Input: part model. Units: mm. Frame: model coordinates. A direction names the side the tool comes from. Coordinates: 2 decimals unless noted, no trailing zeros. Write each loop counter-clockwise with the first axis right and the second up, starting at its lowest first coordinate (ties: lowest second). Pieces come first, ordered by that corner, then holes. Notation, with made-up numbers: M -6,69.25 L 46,69.25 A31 cw 46,107.25 Z; hole C 32.5,80.25 d3. An arc over 180 degrees is marked long. Use one line per item in the form item = value.
from build123d import *

# Parameters (mm, degrees)
F0_W      = 30.5
F0_H      = 22.5
F1_DEPTH  = 6.5
F3_DEPTH  = 3
F4_W      = 7
F4_H      = 4.5
F5_DEPTH  = 3
F6_W      = 6.5
F6_H      = 2.5
F7_DEPTH  = 3.75
F8_W      = 5.8
F8_H      = 1.5
F9_DEPTH  = 0.5
F11_DEPTH = 1
F13_DEPTH = 2.5
F14_W     = 0.5
F14_H     = 0.25
F15_DEPTH = 7
F16_W     = 21.5
F16_H     = 5.5
F17_DEPTH = 1


with BuildPart() as f1:
    # F0 (on Top) → F1 (new body)
    with BuildSketch(Plane.XY):
        Rectangle(F0_W, F0_H)
    extrude(amount=F1_DEPTH)

    # F2 (on face) → F3 (cut)
    with BuildSketch(Plane.XY.offset(6.5)):
        with BuildLine():
            Line((-7.25, 11.25), (-15.25, 11.25))
            Line((-15.25, 11.25), (-15.25, 6.25))
            Line((-15.25, 6.25), (-8.25, 6.25))
            ThreePointArc((-8.25, 6.25), (-7.542893, 6.542893), (-7.25, 7.25))
            Line((-7.25, 7.25), (-7.25, 11.25))
        make_face()
    extrude(amount=-F3_DEPTH, mode=Mode.SUBTRACT)

    # F4 (on face) → F5 (join)
    with BuildSketch(Plane.XY.offset(3.5)):
        with Locations((-11.75, 9)):
            Rectangle(F4_W, F4_H)
    extrude(amount=F5_DEPTH)

    # F6 (on face) → F7 (cut)
    with BuildSketch(Plane(origin=(0, 11.25, 0), x_dir=(-1, 0, 0), z_dir=(0, 1, 0))):
        with Locations((11.75, 5)):
            Rectangle(F6_W, F6_H)
    extrude(amount=-F7_DEPTH, mode=Mode.SUBTRACT)

    # F8 (on face) → F9 (cut)
    with BuildSketch(Plane.XY.offset(6.5)):
        with Locations((-11.75, 10.5)):
            Rectangle(F8_W, F8_H)
    extrude(amount=-F9_DEPTH, mode=Mode.SUBTRACT)

    # F10 (on face) → F11 (cut)
    with BuildSketch(Plane.XY.offset(6.5)):
        with BuildLine():
            Line((10.25, 11.25), (1.75, 11.25))
            Line((1.75, 11.25), (1.75, 8.25))
            ThreePointArc((1.75, 8.25), (2.042893, 7.542893), (2.75, 7.25))
            Line((2.75, 7.25), (9.25, 7.25))
            ThreePointArc((9.25, 7.25), (9.957107, 7.542893), (10.25, 8.25))
            Line((10.25, 8.25), (10.25, 11.25))
        make_face()
    extrude(amount=-F11_DEPTH, mode=Mode.SUBTRACT)

    # F12 (on face) → F13 (join)
    with BuildSketch(Plane(origin=(-15.25, 0, 0), x_dir=(0, -1, 0), z_dir=(-1, 0, 0))):
        with BuildLine():
            Line((10.75, 6.5), (-3.25, 6.5))
            ThreePointArc((-3.25, 6.5), (-3.603553, 6.353553), (-3.75, 6))
            Line((-3.75, 6), (-3.75, 2))
            ThreePointArc((-3.75, 2), (-3.603553, 1.646447), (-3.25, 1.5))
            Line((-3.25, 1.5), (10.75, 1.5))
            ThreePointArc((10.75, 1.5), (11.103553, 1.646447), (11.25, 2))
            Line((11.25, 2), (11.25, 6))
            ThreePointArc((11.25, 6), (11.103553, 6.353553), (10.75, 6.5))
        make_face()
    extrude(amount=F13_DEPTH)

    # F14 (on face) → F15 (join)
    with BuildSketch(Plane(origin=(-17.75, 0, 0), x_dir=(0, -1, 0), z_dir=(-1, 0, 0))):
        with Locations((-2.5, 5.5)):
            Rectangle(F14_W, F14_H)
        with Locations((-2.5, 2.5)):
            Rectangle(F14_W, F14_H)
        with Locations((0, 5.5)):
            Rectangle(F14_W, F14_H)
        with Locations((0, 2.5)):
            Rectangle(F14_W, F14_H)
        with Locations((2.5, 5.5)):
            Rectangle(F14_W, F14_H)
        with Locations((2.5, 2.5)):
            Rectangle(F14_W, F14_H)
        with Locations((5, 5.5)):
            Rectangle(F14_W, F14_H)
        with Locations((5, 2.5)):
            Rectangle(F14_W, F14_H)
        with Locations((7.5, 5.5)):
            Rectangle(F14_W, F14_H)
        with Locations((7.5, 2.5)):
            Rectangle(F14_W, F14_H)
        with Locations((10, 5.5)):
            Rectangle(F14_W, F14_H)
        with Locations((10, 2.5)):
            Rectangle(F14_W, F14_H)
    extrude(amount=F15_DEPTH)

    # F16 (on face) → F17 (cut)
    with BuildSketch(Plane.YZ.offset(15.25)):
        with Locations((0, 3.25)):
            Rectangle(F16_W, F16_H)
    extrude(amount=-F17_DEPTH, mode=Mode.SUBTRACT)


solid = f1.part
(1) First-contact query: pin 1 Ø5 at (x, y) = (-19.5, 4.5) entering from -Z; pin 2 Ø0.8 at (y, z) = (8.5, 5) entering from -X; pin 3 Ø0.6 at (x, y) = (-22.5, -7.5) entering from -Z (3 decimals). Flat tips, straight axial feed; report the tip coordinate or a pass-through.
Computed:
pin_1 = 1.5
pin_2 = -15.25
pin_3 = 2.375
(2) Section query B-B on y = -3.5. Return the cut outline in (x, z).
Computed:
outline = M -17.75,1.5 L -15.25,1.5 L -15.25,0 L 15.25,0 L 15.25,0.5 L 14.25,0.5 L 14.25,6 L 15.25,6 L 15.25,6.5 L -17.75,6.5 Z
(3) Pull-direction query (X, two-part tool) for faces 6 (the flat face through (15, 10.75, 3)), 7 (the flat face through (-7.25, 9, 5)); classes: pulls with the +X half, pulls with the -X half, needs draft (parallel to the pull), parting line crosses it, or undercut.
Computed:
face_6 = needs draft
face_7 = undercut
(4) Line query: probe 1 along Y at (x, z) = (-22, 5.5); probe 2 along X at (y, z) = (7.75, 5.75); probe 3 along X at (y, z) = (-8.5, 1). Output: solid intervals per line, ascending.
Computed:
probe_1 = -10.25 to -9.75, -7.75 to -7.25, -5.25 to -4.75, -2.75 to -2.25, -0.25 to 0.25, 2.25 to 2.75
probe_2 = -15.25 to -15, -8.5 to -8.25, -7.25 to 1.88, 10.12 to 14.25
probe_3 = -15.25 to 14.25
(5) Set-up query: faces 1 (the flat face through (-12, 6.25, 5)), 2 (the flat face through (-12, 9, 6.25)), 3 (the flat face through (15, 0, 6)), 4 (the flat face through (-16, -4, 1.5)), 5 (the cylindrical face through (2.035, 7.551, 6.007)). Return all of +Z, -Z, +X, -X, +Y, -Y with unobstructed straight access to the full face (end or side cutting, diameter ignored); none if empty.
Computed:
face_1 = +Z, -X
face_2 = +Y
face_3 = +X
face_4 = -Z, -X, +Y, -Y
face_5 = +Z, +Y
(6) Section query D-D on x = -20.5. State how many separate pieces and enclosed holes the cut face has, plus the area to 3 significant figures.
Computed:
separate_pieces = 12
enclosed_holes = 0
area = 1.50 mm^2
(7) Section query C-C on x = -10. Return the cut outline in (y, z).
Computed:
outline = M -11.25,0 L 11.25,0 L 11.25,3.75 L 7.5,3.75 L 7.5,6.25 L 9.75,6.25 L 9.75,6.5 L 6.75,6.5 L 6.75,3.5 L 6.25,3.5 L 6.25,6.5 L -11.25,6.5 Z
(8) Section query A-A on z = 4.5. Return the cut outline in (x, y), plus the area to 3 significant figures.
Computed:
outline = M -17.75,-11.25 L 15.25,-11.25 L 15.25,-10.75 L 14.25,-10.75 L 14.25,10.75 L 15.25,10.75 L 15.25,11.25 L -7.25,11.25 L -7.25,7.25 A1 cw -8.25,6.25 L -15.25,6.25 L -15.25,3.75 L -17.75,3.75 Z; M -15.25,6.75 L -8.25,6.75 L -8.25,11.25 L -8.5,11.25 L -8.5,7.5 L -15,7.5 L -15,11.25 L -15.25,11.25 Z
area = 670 mm^2
